Model file for the job. Use its own axes, mm. A direction names the side the tool comes from. Round coordinates to 2 decimals unless told otherwise and drop trailing zeros. Loops run counter-clockwise (first coordinate to the right, second up) from the corner with the lowest first, then second, coordinate; pieces in that order, holes last. Notation, with made-up numbers: M -36,56.25 L -20,56.25 A18 cw -20,85.25 Z; hole C -23,25.25 d1. An arc over 180 degrees is marked long. Use a Markdown table: item, result. Add a question column.
Q1. Cut at B-B (z = 1). Give the cut face in (x, y), plus the area to 3 significant figures.
Q2. Pin check, flat tips, straight feed: pin 1 (17.5 mm diameter, centred on x = 18.5, y = -15.5, fed in from +Z); pin 2 (2 mm diameter, centred on y = -8, z = 5, fed in from -X); pin 3 (5.5 mm diameter, centred on x = 1, z = 5, fed in from +Y). Stop position of each tip, or through.
Q3. Mould opens along Y. For faces 1 (the face through (22, 0, 3)), 2 (the face through (15, -5, 3)), 3 (the face through (22, 5, 3)) say: +Y half, -Y half, draft (parallel to the pull), parting line (faces both ways), or undercut.
Q4. Cut at D-D (z = 4). Give the cut face in (x, y), plus the area to 3 significant figures.
Q5. Probe line 1 (Y direction, x = 22.5, z = 3.75); line 2 (Y direction, x = 22.5, z = 2.25); line 3 (Z direction, x = 28, y = -27). List the from-to ranges inside material, lowest first. Write a range as from..to.
Q6. Tool access for faces 4 (the face through (13, -30, 3)), 5 (the face through (5, -15, 3)), 6 (the face through (19.5, 0.1, 10)): list every direction of +Z, -Z, +X, -X, +Y, -Y with a clear straight run to the whole face (end or side of a thin tool).
Q7. Cut at C-C (x = 22.5). Give the cut face in (y, z).
Q8. Cut at A-A (y = -22.5). Give the cut face in (x, z).
from build123d import *

# Parameters (mm, degrees)
SKETCH008_R     = 2.25
PAD005_DEPTH    = 7
SKETCH009_R     = 3
POCKET003_DEPTH = 30.001
SKETCH010_R     = 3
POCKET004_DEPTH = 30.001
SKETCH011_R     = 3
PAD006_DEPTH    = 6


with BuildPart() as part:
    # Sketch008 → Pad005 (new body)
    with BuildSketch(Plane.XY):
        Polygon((-5, -30), (-5, -15), (15, -15), (15, 5), (30, 5), (30, -30), align=None)
        with Locations((22.5, -22.5)):
            Circle(SKETCH008_R, mode=Mode.SUBTRACT)
    extrude(amount=PAD005_DEPTH)

    # Sketch009 → Pocket003 (cut, through all)
    with BuildSketch(Plane.XZ):
        Circle(SKETCH009_R)
    extrude(amount=POCKET003_DEPTH, mode=Mode.SUBTRACT)

    # Sketch010 → Pocket004 (cut, through all)
    with BuildSketch(Plane.YZ):
        Circle(SKETCH010_R)
    extrude(amount=POCKET004_DEPTH, mode=Mode.SUBTRACT)

    # Sketch011 → Pad006 (join)
    with BuildSketch(Plane.XY.offset(7)):
        with Locations((22.5, 0)):
            Circle(SKETCH011_R)
    extrude(amount=PAD006_DEPTH)


solid = part.part
Checked values:
| question | item | result |
|---|---|---|
| 1 | outline | M -5,-30 L -2.83,-30 L -2.83,-15 L -5,-15 Z; M 2.83,-30 L 30,-30 L 30,-2.83 L 15,-2.83 L 15,-15 L 2.83,-15 Z; M 15,2.83 L 30,2.83 L 30,5 L 15,5 Z; hole C 22.5,-22.5 d4.5 |
| 1 | area | 639 mm^2 |
| 2 | pin 1 | stops at z = 7 |
| 2 | pin 2 | stops at x = 15 |
| 2 | pin 3 | stops at y = -15 |
| 3 | face 1 | undercut |
| 3 | face 2 | draft |
| 3 | face 3 | +Y half |
| 4 | outline | M -5,-30 L 30,-30 L 30,5 L 15,5 L 15,-15 L -5,-15 Z; hole C 22.5,-22.5 d4.5 |
| 4 | area | 809 mm^2 |
| 5 | line 1 | y = -30..-24.75, -20.25..5 |
| 5 | line 2 | y = -30..-24.75, -20.25..-1.98, 1.98..5 |
| 5 | line 3 | z = 0..7 |
| 6 | face 4 | +Z, -Z, +X, -X, -Y |
| 6 | face 5 | +Z, -Z, -X, +Y |
| 6 | face 6 | +Z |
| 7 | outline | M -30,0 L -24.75,0 L -24.75,7 L -30,7 Z; M -20.25,0 L -3,0 A3 cw 3,0 L 5,0 L 5,7 L 3,7 L 3,13 L -3,13 L -3,7 L -20.25,7 Z |
| 8 | outline | M -5,0 L -3,0 A3 cw 3,0 L 20.25,0 L 20.25,7 L -5,7 Z; M 24.75,0 L 30,0 L 30,7 L 24.75,7 Z |
